Design review of the part built by this model. Coordinates are the model's own, in mm. A direction names the side the tool comes from. Round coordinates to 2 decimals unless told otherwise and drop trailing zeros. Order: outer loops, then holes, each group sorted by start corner. A loop starts at its lowest first (then second) coordinate and runs counter-clockwise, first axis right, second up.
from build123d import *

# Parameters (mm, degrees)
SKETCH_1_W          = 50
SKETCH_1_H          = 5
EXTRUDE_1_DEPTH     = 20
EXTRUDE_2_DEPTH     = 20
SKETCH_3_R          = 2.5
CUT_EXTRUDE_1_DEPTH = 20


with BuildPart() as part:
    # 草图1 → 凸台-拉伸1 (new body)
    with BuildSketch(Plane.XY):
        with Locations((0, 2.5)):
            Rectangle(SKETCH_1_W, SKETCH_1_H)
    extrude(amount=EXTRUDE_1_DEPTH)

    # 草图2 → 凸台-拉伸2 (add)
    with BuildSketch(Plane.XY.offset(20)):
        with BuildLine():
            Line((-5, 10), (-5, 5))
            Line((-5, 5), (5, 5))
            Line((5, 5), (5, 10))
            ThreePointArc((5, 10), (0, 15), (-5, 10))
        make_face()
    extrude(amount=-EXTRUDE_2_DEPTH)

    # 草图3 → 切除-拉伸1 (cut)
    with BuildSketch(Plane.XY.offset(20)):
        with Locations((0, 10)):
            Circle(SKETCH_3_R)
    extrude(amount=-CUT_EXTRUDE_1_DEPTH, mode=Mode.SUBTRACT)


solid = part.part
1) The part is to be moulded in two halves that separate along X. For faces 1 (the face through (0, 3, 0)), 2 (the face through (-25, 2, 10)), 3 (the face through (25, 2, 10)), 4 (the face through (-0.54, 7.56, 10.14)), say which applies: released by +X, released by -X, zero draft, split by the parting line, or undercut.
Results:
face 1: zero draft
face 2: released by -X
face 3: released by +X
face 4: undercut
2) Take a section at C-C on y = 8.75. Give the boundary of the cut face in (x, z), plus the area to 3 significant figures.
Results:
outline: (-5, 0) - (-2.17, 0) - (-2.17, 20) - (-5, 20) - close; (2.17, 0) - (5, 0) - (5, 20) - (2.17, 20) - close
area: 113 mm2
3) Take a section at A-A on z = 14. Give the boundary of the cut face in (x, y), plus the area to 3 significant figures.
Results:
outline: (-25, 0) - (25, 0) - (25, 5) - (5, 5) - (5, 10) arc R5 ccw to (-5, 10) - (-5, 5) - (-25, 5) - close; hole circle Ø5 at (0, 10)
area: 320 mm2
4) For faces 5 (the face through (0, 15, 10)), 6 (the face through (5, 7, 10)), 7 (the face through (-5, 8, 10)), list the 3-axis set-ups (+Z, -Z, +X, -X, +Y, -Y) from which the entire face can be reached by the end or side of a thin tool; tool diameter is ignored.
Results:
face 5: +Z, -Z, +Y
face 6: +Z, -Z, +X, +Y
face 7: +Z, -Z, -X, +Y
5) Clearance check with flat-ended pins moving along their axes: P1, Ø2.5, axis at y = 7.5, z = 5.5, coming from the +X side; P2, Ø5, axis at x = -14, z = 2.5, coming from the +Y side; P3, Ø1.5, axis at y = 7.5, z = 14.5, coming from the -X side. State where each tip first meets the part, or that it passes through.
Results:
P1: stops at x = 5
P2: stops at y = 5
P3: stops at x = -5
6) To check wall thickness, follow line 1 along Y through (x, z) = (0, 6.75); line 2 along Y through (x, z) = (19, 17.75); line 3 along X through (y, z) = (6.75, 3.5). State the ranges of each line that lie inside material, in increasing order.
Results:
line 1: y = 0 to 7.5, 12.5 to 15
line 2: y = 0 to 5
line 3: x = -5 to 5
7) Take a section at D-D on x = -16.5. Give the boundary of the cut face in (y, z), plus the area to 3 significant figures.
Results:
outline: (0, 0) - (5, 0) - (5, 20) - (0, 20) - close
area: 100 mm2
8) Take a section at B-B on x = 0. Give the boundary of the cut face in (y, z).
Results:
outline: (0, 0) - (7.5, 0) - (7.5, 20) - (0, 20) - close; (12.5, 0) - (15, 0) - (15, 20) - (12.5, 20) - close
